Geometry check sheet. Reference: the model listing, model coordinates, mm. Face numbers are marked on the shaded views. A direction names the side the tool comes from. Coordinates: 2 decimals unless noted, no trailing zeros. Write each loop counter-clockwise with the first axis right and the second up, starting at its lowest first coordinate (ties: lowest second). Pieces come first, ordered by that corner, then holes. Notation, with made-up numbers: M 6.25,8.5 L 58.25,8.5 A27 cw 58.25,25.5 Z; hole C 84.25,26.25 d8. An arc over 180 degrees is marked long. Write item = value, one per line. Start each with the question number.
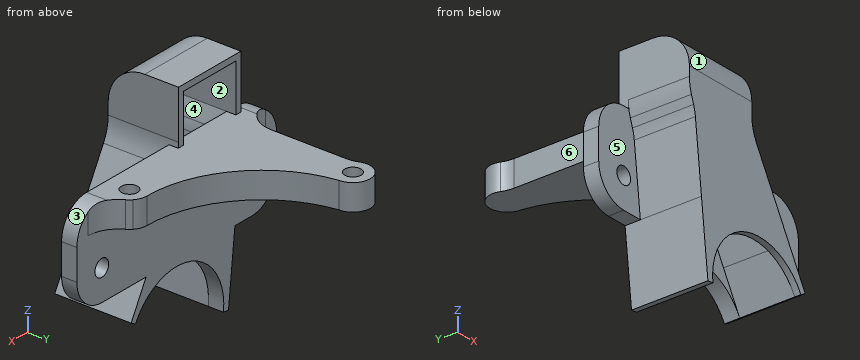
```python
from build123d import *

# Parameters (mm, degrees)
SKETCH1_W           = 80
SKETCH1_H           = 30
SKETCH1_R           = 2.75
BOSS_EXTRUDE1_DEPTH = 5
SKETCH2_W           = 51.3
SKETCH2_H           = 8.5
BOSS_EXTRUDE2_DEPTH = 50
SKETCH3_R           = 2.665
CUT_EXTRUDE1_DEPTH  = 8
CUT_EXTRUDE2_REACH  = 76.33
BOSS_EXTRUDE3_DEPTH = 8.5
FILLET1_START       = 6.5
FILLET1_DEPTH       = 8.5
FILLET2_R           = 10
BOSS_EXTRUDE5_DEPTH = 5
BOSS_EXTRUDE6_DEPTH = 20
BOSS_EXTRUDE7_DEPTH = 20
CUT_EXTRUDE3_DEPTH  = 20
BOSS_EXTRUDE8_DEPTH = 3
FILLET4_START       = -20
FILLET4_DEPTH       = 20
FILLET4_2_DEPTH     = 4
FILLET4_3_DEPTH     = 23
BOSS_EXTRUDE9_DEPTH = 2
FILLET5_R           = 12


with BuildPart() as part:
    # Sketch1 → Boss-Extrude1 (new body)
    with BuildSketch(Plane(origin=(0, 0, 0), x_dir=(1, 0, 0), z_dir=(0, 1, 0))):
        Rectangle(SKETCH1_W, SKETCH1_H)
        with Locations(Location((30, 5, 0), (0, 0, 270))):
            Circle(SKETCH1_R, mode=Mode.SUBTRACT)
        with Locations(Location((-30, 5, 0), (0, 0, 270))):
            Circle(SKETCH1_R, mode=Mode.SUBTRACT)
    extrude(amount=BOSS_EXTRUDE1_DEPTH)

    # Sketch2 → Boss-Extrude2 (add)
    with BuildSketch(Plane(origin=(0, 5, 0), x_dir=(1, 0, 0), z_dir=(0, 1, 0))):
        with Locations((0, -10.75)):
            Rectangle(SKETCH2_W, SKETCH2_H)
    extrude(amount=BOSS_EXTRUDE2_DEPTH)

    # Sketch3 → Cut-Extrude1 (cut)
    with BuildSketch(Plane.XY.offset(15)):
        with Locations((21.85, 7.4)):
            Circle(SKETCH3_R)
        with Locations((-21.15, 45.4)):
            Circle(SKETCH3_R)
    extrude(amount=-CUT_EXTRUDE1_DEPTH, mode=Mode.SUBTRACT)

    # Sketch5 → Cut-Extrude2 (cut, up to next)
    with BuildSketch(Plane.XY.offset(15), mode=Mode.PRIVATE) as cut_extrude2_sk1:
        with BuildLine():
            ThreePointArc((-15.485, 45.4), (-2.845416832, 22.272479127), (21.85, 13.065))
            ThreePointArc((21.85, 13.065), (23.886047867, 12.68646707), (25.65, 11.601455105))
            Line((25.65, 11.601455105), (25.65, 55))
            Line((25.65, 55), (-25.65, 55))
            Line((-25.65, 55), (-25.65, 48.841253405))
            ThreePointArc((-25.65, 48.841253405), (-19.333447634, 50.765851517), (-15.485, 45.4))
        make_face()
    cut_extrude2_tool1 = extrude(cut_extrude2_sk1.sketch, amount=-CUT_EXTRUDE2_REACH, mode=Mode.PRIVATE) & part.part
    add(cut_extrude2_tool1.solids().sort_by_distance((6.645392, 37.171167, 15))[0], mode=Mode.SUBTRACT)

    # Sketch5<3> → Boss-Extrude3 (add)
    with BuildSketch(Plane.XY.offset(15)):
        with BuildLine():
            Line((25.65, 5), (26.981493447, 5))
            ThreePointArc((26.981493447, 5), (27.380015162, 6.170708615), (27.515, 7.4))
            ThreePointArc((27.515, 7.4), (27.027799967, 9.698393461), (25.65, 11.601455105))
            Line((25.65, 11.601455105), (25.65, 5))
        make_face()
        with BuildLine():
            ThreePointArc((-25.65, 48.841253405), (-26.815, 45.4), (-25.65, 41.958746595))
            Line((-25.65, 41.958746595), (-25.65, 48.841253405))
        make_face()
    extrude(amount=-BOSS_EXTRUDE3_DEPTH)

    # Fillet1: read off the stored shape, not the designer's step
    # Fillet1 outline → Fillet1 (add)
    with BuildSketch(Plane.XY.offset(FILLET1_START)):
        with BuildLine():
            ThreePointArc((-26.393696138, 43.256200613), (-25.837685324, 41.400248446), (-25.65, 39.471912197))
            Line((-25.65, 39.471912197), (-25.65, 41.958746595))
            ThreePointArc((-25.65, 41.958746595), (-26.064849981, 42.582825057), (-26.393696138, 43.256200613))
        make_face()
        with BuildLine():
            Line((-35.65, 5), (-25.65, 5))
            Line((-25.65, 5), (-25.65, 15))
            ThreePointArc((-25.65, 15), (-28.578932188, 7.928932188), (-35.65, 5))
        make_face()
        with BuildLine():
            ThreePointArc((35.547891261, 5), (30.474223926, 6.382697651), (26.803626173, 10.148420045))
            ThreePointArc((26.803626173, 10.148420045), (27.511622265, 7.595597351), (26.981493447, 5))
            Line((26.981493447, 5), (35.547891261, 5))
        make_face()
    extrude(amount=FILLET1_DEPTH)

    # Fillet2
    fillet2_edges = [part.edges().sort_by_distance(p)[0] for p in [
        (40, 2.5, 15),
        (40, 2.5, -15),
        (-40, 2.5, -15),
        (-40, 2.5, 15),
    ]]
    fillet(fillet2_edges, radius=FILLET2_R)

    # Sketch7 → Boss-Extrude5 (add)
    with BuildSketch(Plane.XZ):
        with BuildLine():
            Line((16.505683811, -26.744235317), (9.991112457, -15))
            Line((9.991112457, -15), (-21.314804171, -15))
            Line((-21.314804171, -15), (-18.759427627, -37.985545514))
            ThreePointArc((-18.759427627, -37.985545514), (-5.732504168, -17.916562593), (16.505683811, -26.744235317))
        make_face()
        Polygon((-18.759427627, -37.985545514), (-21.314804171, -15), (-23.327125696, -15), (-20.747181548, -38.206530469), align=None)
        Polygon((12.278203403, -15), (9.991112457, -15), (16.505683811, -26.744235317), (18.25463044, -25.774088066), align=None)
    extrude(amount=-BOSS_EXTRUDE5_DEPTH)

    # Sketch7<6> → Boss-Extrude6 (add)
    with BuildSketch(Plane.XZ):
        Polygon((-4.362909054, 15), (-6.65, 15), (9.991112457, -15), (12.278203403, -15), align=None)
        Polygon((12.278203403, -15), (9.991112457, -15), (16.505683811, -26.744235317), (18.25463044, -25.774088066), align=None)
        Polygon((-21.314804171, -15), (-24.650000035, 15), (-26.662321559, 15), (-26.637753956, 14.779015045), (-23.327125696, -15), align=None)
        Polygon((-18.759427627, -37.985545514), (-21.314804171, -15), (-23.327125696, -15), (-20.747181548, -38.206530469), align=None)
    extrude(amount=BOSS_EXTRUDE6_DEPTH)

    # Sketch8 → Boss-Extrude7 (add)
    with BuildSketch(Plane.XZ):
        Polygon((-5.15, 30.5), (-5.15, 22), (-5.15, 15), (-4.362909054, 15), (-3.15, 15), (-3.15, 22), (-3.15, 32.5), (-28.15, 32.5), (-28.15, 22), (-28.15, 15), (-25.9441307, 8.539891907), (-26.662321559, 15), (-26.15, 15), (-26.15, 22), (-26.15, 30.5), align=None)
        Polygon((-3.15, 15), (-4.362909054, 15), (-3.15, 12.813411109), align=None)
    extrude(amount=BOSS_EXTRUDE7_DEPTH)

    # Sketch8<3> → Cut-Extrude3 (cut)
    with BuildSketch(Plane.XZ):
        Polygon((-23.925860843, 8.48638681), (-24.650000035, 15), (-26.15, 15), align=None)
        Polygon((-6.65, 15), (-5.15, 15), (-5.15, 12.295853861), align=None)
    extrude(amount=CUT_EXTRUDE3_DEPTH, mode=Mode.SUBTRACT)

    # Sketch9 → Boss-Extrude8 (add)
    with BuildSketch(Plane(origin=(0, 0, 0), x_dir=(1, 0, 0), z_dir=(0, 1, 0))):
        Polygon((-3.15, -32.5), (-3.15, -15), (-5.15, -15), (-5.15, -30.5), (-26.15, -30.5), (-26.15, -15), (-28.15, -15), (-28.15, -32.5), align=None)
    extrude(amount=BOSS_EXTRUDE8_DEPTH)

    # Fillet4: read off the stored shape, not the designer's step
    # Fillet4 outline → Fillet4 (cut)
    with BuildSketch(Plane(origin=(0, 0, 0), x_dir=(1, 0, 0), z_dir=(0, 1, 0)).offset(FILLET4_START)):
        with BuildLine():
            ThreePointArc((-5.15, -16.177533225), (-4.671647561, -12.419641247), (-3.267099718, -8.901428842))
            Line((-3.267099718, -8.901428842), (-5.15, -12.295853861))
            Line((-5.15, -12.295853861), (-5.15, -16.177533225))
        make_face()
        with BuildLine():
            ThreePointArc((-28.15, -17.490360897), (-27.947447955, -15.033628513), (-27.345262132, -12.643244951))
            Line((-27.345262132, -12.643244951), (-28.15, -15))
            Line((-28.15, -15), (-28.15, -17.490360897))
        make_face()
        with BuildLine():
            ThreePointArc((-23.744211533, -6.852455992), (-24.013520151, -8.466795288), (-24.457103806, -10.042184774))
            Line((-24.457103806, -10.042184774), (-23.925860843, -8.48638681))
            Line((-23.925860843, -8.48638681), (-23.744211533, -6.852455992))
        make_face()
    extrude(amount=FILLET4_DEPTH, mode=Mode.SUBTRACT)

    # Fillet4 2 outline → Fillet4 2 (cut)
    with BuildSketch(Plane(origin=(0, 0, 0), x_dir=(1, 0, 0), z_dir=(0, 1, 0))):
        with BuildLine():
            Line((-5.15, -15), (-5.15, -16.177533225))
            ThreePointArc((-5.15, -16.177533225), (-5.138422804, -15.588311844), (-5.103709089, -15))
            Line((-5.103709089, -15), (-5.15, -15))
        make_face()
    extrude(amount=FILLET4_2_DEPTH, mode=Mode.SUBTRACT)

    # Fillet4 3 outline → Fillet4 3 (add)
    with BuildSketch(Plane(origin=(0, 0, 0), x_dir=(1, 0, 0), z_dir=(0, 1, 0)).offset(FILLET4_START)):
        with BuildLine():
            ThreePointArc((-25.76248139, -6.905961089), (-26.031790008, -8.520300385), (-26.475373663, -10.095689871))
            Line((-26.475373663, -10.095689871), (-25.9441307, -8.539891907))
            Line((-25.9441307, -8.539891907), (-25.76248139, -6.905961089))
        make_face()
        with BuildLine():
            Line((-3.15, -12.813411109), (-3.15, -16.695090474))
            ThreePointArc((-3.15, -16.695090474), (-2.671647561, -12.937198496), (-1.267099718, -9.41898609))
            Line((-1.267099718, -9.41898609), (-3.15, -12.813411109))
        make_face()
    extrude(amount=FILLET4_3_DEPTH)

    # Sketch10 → Boss-Extrude9 (add)
    with BuildSketch(Plane.XZ.offset(20)):
        with BuildLine():
            ThreePointArc((16.505683811, -26.744235317), (-5.732504168, -17.916562593), (-18.759427627, -37.985545514))
            Line((-18.759427627, -37.985545514), (-23.744211533, 6.852455992))
            ThreePointArc((-23.744211533, 6.852455992), (-24.013520151, 8.466795288), (-24.457103806, 10.042184774))
            Line((-24.457103806, 10.042184774), (-26.15, 15))
            Line((-26.15, 15), (-26.15, 30.5))
            Line((-26.15, 30.5), (-5.15, 30.5))
            Line((-5.15, 30.5), (-5.15, 16.177533225))
            ThreePointArc((-5.15, 16.177533225), (-4.671647561, 12.419641247), (-3.267099718, 8.901428842))
            Line((-3.267099718, 8.901428842), (16.505683811, -26.744235317))
        make_face()
        with BuildLine():
            Line((-26.15, 30.5), (-5.15, 30.5))
            Line((-5.15, 30.5), (-5.15, 16.177533225))
            ThreePointArc((-5.15, 16.177533225), (-4.671647561, 12.419641247), (-3.267099718, 8.901428842))
            Line((-3.267099718, 8.901428842), (16.505683811, -26.744235317))
            Line((16.505683811, -26.744235317), (18.25463044, -25.774088066))
            Line((18.25463044, -25.774088066), (-1.267099718, 9.41898609))
            ThreePointArc((-1.267099718, 9.41898609), (-2.671647561, 12.937198496), (-3.15, 16.695090474))
            Line((-3.15, 16.695090474), (-3.15, 32.5))
            Line((-3.15, 32.5), (-28.15, 32.5))
            Line((-28.15, 32.5), (-28.15, 17.490360897))
            ThreePointArc((-28.15, 17.490360897), (-27.947447955, 15.033628513), (-27.345262132, 12.643244951))
            Line((-27.345262132, 12.643244951), (-26.475373663, 10.095689871))
            ThreePointArc((-26.475373663, 10.095689871), (-26.031790008, 8.520300385), (-25.76248139, 6.905961089))
            Line((-25.76248139, 6.905961089), (-20.747181548, -38.206530469))
            Line((-20.747181548, -38.206530469), (-18.759427627, -37.985545514))
            Line((-18.759427627, -37.985545514), (-23.744211533, 6.852455992))
            ThreePointArc((-23.744211533, 6.852455992), (-24.013520151, 8.466795288), (-24.457103806, 10.042184774))
            Line((-24.457103806, 10.042184774), (-26.15, 15))
            Line((-26.15, 15), (-26.15, 30.5))
        make_face()
    extrude(amount=-BOSS_EXTRUDE9_DEPTH)

    # Fillet5
    fillet5_edges = [part.edges().sort_by_distance(p)[0] for p in [
        (-15.65, -20, 32.5),
        (-15.65, -18, 30.5),
    ]]
    fillet(fillet5_edges, radius=FILLET5_R)


solid = part.part
```
Q1. Draft check along X on the marked faces 1, 2 and 3. Enter one of: pulls with the +X half, pulls with the -X half, needs draft (parallel to the pull), parting line crosses it, or undercut.
Q2. Cross-section at D-D on y = 33. Enter the section's corners in (x, z).
Q3. Cross-section at C-C on z = -13. Enter the section's corners in (x, y).
Q4. Gauge pin test, flat ends, axial feed: pin 1 (6 mm diameter, centred on x = -21, y = 46.5, fed in from +Z); pin 2 (10 mm diameter, centred on x = 20.5, z = -5, fed in from +Y); pin 3 (24 mm diameter, centred on x = 22.5, z = 6, fed in from -Y); pin 4 (4.5 mm diameter, centred on x = 30, z = -5, fed in from -Y). Record the tip position at first contact, or that the pin passes through.
Q5. Cross-section at A-A on y = -13.5. Enter the section's corners in (x, z).
Q6. Cross-section at B-B on z = 22.5. Enter the section's corners in (x, y).
Q7. Scan lines: L1, parallel to X at y = 2.1, z = -5; L2, parallel to Y at x = -0.5, z = -17; L3, parallel to Y at x = -21.15, z = 12.25 (3 decimals). Record each from-to range of solid material in increasing order.
Q8. Set-up check for the marked faces 4, 5 and 6: record each of +Z, -Z, +X, -X, +Y, -Y from which the full face is reachable in a straight line by a thin tool's end or side.
Values found:
q1.face_1 = needs draft
q1.face_2 = undercut
q1.face_3 = pulls with the +X half
q2.outline = M -25.65,6.5 L -11.41,6.5 L -11.41,15 L -25.65,15 Z
q3.outline = M -36,0 L -23.55,0 L -23.55,-20 L 11.17,-20 L 11.17,0 L 36,0 L 36,5 L -36,5 Z; hole M -21.54,-18 L 8.88,-18 L 8.88,0 L -21.54,0 Z
q4.pin_1 = 15
q4.pin_2 = 5
q4.pin_3 = 0
q4.pin_4 = through
q5.outline = M -28.15,17.49 A15 ccw -27.35,12.64 L -26.48,10.1 A15 cw -25.76,6.91 L -20.75,-38.21 L -18.76,-37.99 L -23.74,6.85 A15 ccw -24.46,10.04 L -26.15,15 L -26.15,27.87 L -5.15,27.87 L -5.15,16.18 A15 ccw -3.27,8.9 L 16.51,-26.74 L 18.25,-25.77 L -1.27,9.42 A15 cw -3.15,16.7 L -3.15,31.17 L -28.15,31.17 Z
q6.outline = M -28.15,-19.83 L -3.15,-19.83 L -3.15,3 L -5.15,3 L -5.15,-17.31 L -26.15,-17.31 L -26.15,3 L -28.15,3 Z
q7.L1 = -40 to -32.75, -27.25 to 27.25, 32.75 to 40
q7.L2 = -20 to -18, 0 to 5
q7.L3 = -20 to -18, 0 to 42.735, 48.065 to 51.065
q8.face_4 = none
q8.face_5 = -Z, -X, -Y
q8.face_6 = +Z, -Z, -X
